Verification items for the finished model (mm, model axes). A direction names the side the tool comes from. Coordinates: 2 decimals unless noted, no trailing zeros. Write each loop counter-clockwise with the first axis right and the second up, starting at its lowest first coordinate (ties: lowest second). Pieces come first, ordered by that corner, then holes. Notation, with made-up numbers: (-17.5, 60.25) -> (23.5, 60.25) arc R27 ccw to (23.5, 98.25) -> close; hole circle Ø4 at (38, -3). An arc over 180 degrees is marked (long way). Use a Markdown table: item, result. Add a question column.
from build123d import *

# Parameters (mm, degrees)
F0_W      = 65.485179
F0_H      = 37.281514
F1_DEPTH  = 50.8
F2_DEPTH  = 25.4
F4_DEPTH  = 50.8
F5_DEPTH  = 25.4
F6_W      = 65.805174
F6_H      = 12.657734
F7_DEPTH  = 38.1
F8_R      = 4.088861
F8_R_2    = 4.00946
F8_R_3    = 3.015148
F8_R_4    = 3.207559
F9_DEPTH  = 50.8
F10_R     = 4.296348
F10_R_2   = 4.287756
F11_DEPTH = 25.4


with BuildPart() as f1:
    # F0 (on Front) → F1 (new body)
    with BuildSketch(Plane.XZ):
        with Locations((-32.74259, 3.37556)):
            Rectangle(F0_W, F0_H)
        Polygon((19.307569, 12.089744), (0, 22.016317), (0, -15.265197), (0, -24.720937), (19.307569, -24.720937), (19.307569, -15.265197), align=None)
    extrude(amount=F1_DEPTH)

    # F0 (on Front) → F2 (join)
    with BuildSketch(Plane.XZ):
        Polygon((72.358251, -15.265197), (19.307569, 12.089744), (19.307569, -15.265197), (64.418688, -15.265197), align=None)
    extrude(amount=F2_DEPTH)

    # F3 (on Front) → F4 (join)
    with BuildSketch(Plane.XZ):
        Polygon((0, 22.467867), (-65.891236, 22.467867), (-65.404281, -15.514851), (0, -15.514851), align=None)
        Polygon((19.326396, 12.241751), (0, 22.467867), (0, -15.514851), (0, -24.767056), (19.326396, -24.929374), (19.326396, -15.677169), align=None)
    extrude(amount=F4_DEPTH)

    # F0 (on Front) → F5 (join)
    with BuildSketch(Plane.XZ):
        Polygon((72.358251, -15.265197), (19.307569, 12.089744), (19.307569, -15.265197), (64.418688, -15.265197), align=None)
    extrude(amount=F5_DEPTH)

    # F6 (on Top) → F7 (cut)
    with BuildSketch(Plane.XY):
        with Locations((-32.902587, -25.323051)):
            Rectangle(F6_W, F6_H)
    extrude(amount=F7_DEPTH, mode=Mode.SUBTRACT)

    # F8 (on Top) → F9 (cut)
    with BuildSketch(Plane.XY):
        with Locations((29.517371, -19.660087)):
            Circle(F8_R)
        with Locations((29.071776, -8.137451)):
            Circle(F8_R_2)
        with Locations((55.278175, -19.761529)):
            Circle(F8_R_3)
        with Locations((54.863308, -8.436291)):
            Circle(F8_R_4)
    extrude(amount=F9_DEPTH, mode=Mode.SUBTRACT)

    # F10 (on face) → F11 (cut)
    with BuildSketch(Plane(origin=(8.979881, 0, 17.415091), x_dir=(0.888799, 0, -0.458298), z_dir=(0.458298, 0, 0.888799))):
        with Locations((45.114581, -19.458767)):
            Circle(F10_R)
        with Locations((44.607103, -8.562293)):
            Circle(F10_R_2)
    extrude(amount=-F11_DEPTH, mode=Mode.SUBTRACT)


solid = f1.part
1) Cross-section at D-D on z = 19. Record the boundary of the cut face in (x, y), then the cut area to 3 significant figures.
2) Thickness scan on L1, parallel to Y at x = -52, z = 4; L2, parallel to Z at x = -6.5, y = -8; L3, parallel to X at y = -20.5, z = -8. Record the ranges inside material, lowest first.
3) Cross-section at A-A on y = -43. Record the boundary of the cut face in (x, z).
4) Set-up check for faces 1 (the face through (45, -13, -15.265)), 2 (the face through (0, -25, -20)), 3 (the face through (25.066, -7.961, 3.516)): record each of +Z, -Z, +X, -X, +Y, -Y from which the full face is reachable in a straight line by a thin tool's end or side.
5) Cross-section at B-B on y = -28. Record the boundary of the cut face in (x, z) (3 decimals), then the cut area to 3 significant figures.
6) Release check for a two-part mould opening along X. For faces 4 (the face through (-24, -50.8, 4)), 5 (the face through (0, -25, 11)), 6 (the face through (-33, -31.652, 11)), 7 (the face through (46.21, -12.52, -1.78)) record: released by +X, released by -X, zero draft, split by the parting line, or undercut.
7) Cross-section at C-C on x = -39. Record the boundary of the cut face in (y, z), then the cut area to 3 significant figures.
8) Gauge pin test, flat ends, axial feed: pin 1 (9 mm diameter, centred on x = 27.5, y = -6.5, fed in from +Z); pin 2 (11 mm diameter, centred on y = -31.5, z = -12, fed in from +X); pin 3 (6.5 mm diameter, centred on x = -44.5, y = -27, fed in from +Z); pin 4 (6 mm diameter, centred on x = 46, z = -1.5, fed in from +Y). Record the tip position at first contact, or that the pin passes through.
Returned:
| question | item | result |
|---|---|---|
| 1 | outline | (-65.85, -50.8) -> (6.55, -50.8) -> (6.55, 0) -> (-65.85, 0) -> close; hole (-65.81, -31.65) -> (0, -31.65) -> (0, -18.99) -> (-65.81, -18.99) -> close |
| 1 | area | 2,850 mm² |
| 2 | L1 | y = -50.8 to -31.65, -18.99 to 0 |
| 2 | L2 | z = -15.51 to 22.47 |
| 2 | L3 | x = -65.5 to 41.94, 51.32 to 58.27 |
| 3 | outline | (-65.89, 22.47) -> (-65.49, -9.2) -> (-65.49, -15.27) -> (-65.41, -15.27) -> (-65.4, -15.51) -> (0, -15.51) -> (0, -24.77) -> (19.33, -24.93) -> (19.33, 12.24) -> (0, 22.47) -> close |
| 4 | face 1 | -Z, +X, +Y, -Y |
| 4 | face 2 | -Z, -X, +Y, -Y |
| 4 | face 3 | +Z |
| 5 | outline | (-65.891, 22.468) -> (-65.805, 15.755) -> (-65.805, 22.468) -> close; (-65.603, 0) -> (-65.485, -9.205) -> (-65.485, -15.265) -> (-65.407, -15.265) -> (-65.404, -15.515) -> (0, -15.515) -> (0, -24.767) -> (19.326, -24.929) -> (19.326, 12.242) -> (0, 22.468) -> (0, 0) -> close |
| 5 | area | 1,830 mm² |
| 6 | face 4 | zero draft |
| 6 | face 5 | undercut |
| 6 | face 6 | undercut |
| 6 | face 7 | released by +X |
| 7 | outline | (-50.8, -15.51) -> (0, -15.51) -> (0, 22.47) -> (-18.99, 22.47) -> (-18.99, 0) -> (-31.65, 0) -> (-31.65, 22.47) -> (-50.8, 22.47) -> close |
| 7 | area | 1,650 mm² |
| 8 | pin 1 | stops at z = 10.19 |
| 8 | pin 2 | stops at x = 19.33 |
| 8 | pin 3 | stops at z = 0 |
| 8 | pin 4 | stops at y = 0 |
